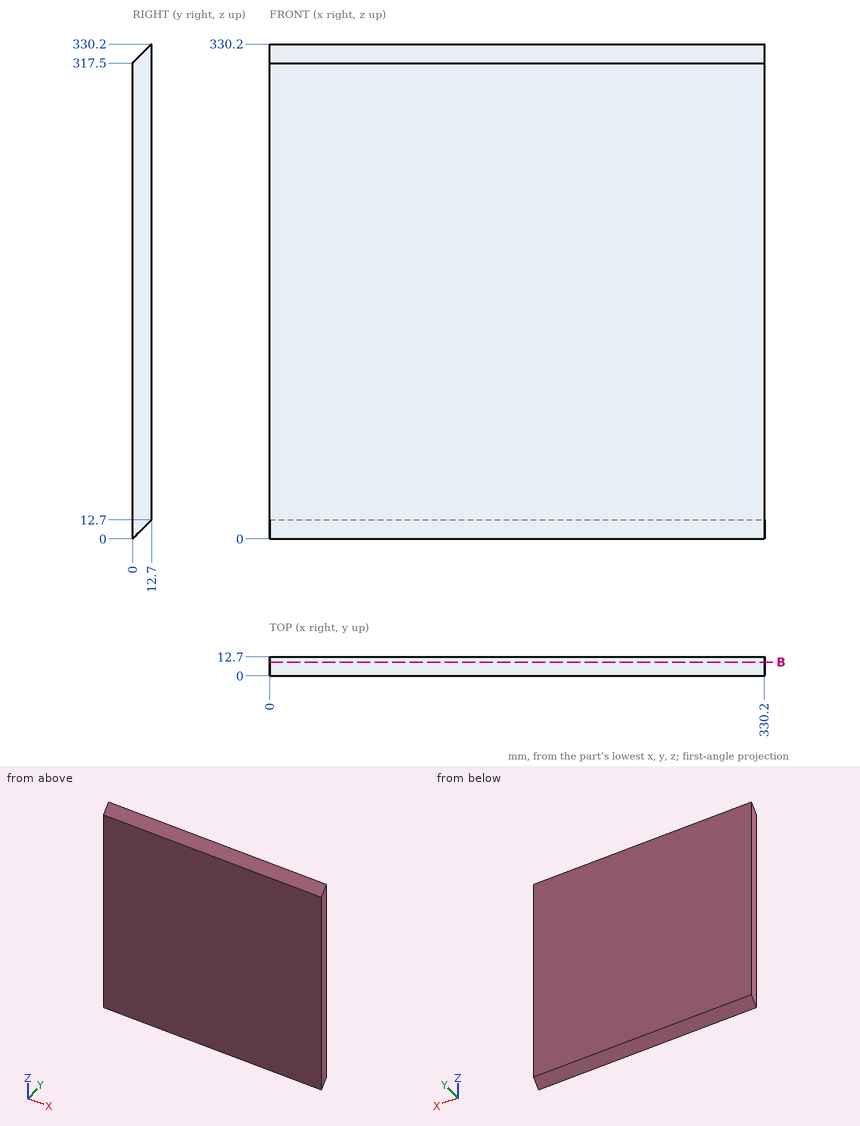
For this review, use the dimensioned drawing (mm, ordinates from the lowest corner) and the shaded views. Coordinates: 2 decimals unless noted, no trailing zeros. Order: outer loops, then holes, each group sorted by start corner. A loop starts at its lowest first (then second) coordinate and runs counter-clockwise, first axis right, second up. Notation, with made-up numbers: M 89.5,87.25 L 130.5,87.25 A23 cw 130.5,112.25 Z; hole C -16,35 d6. An arc over 180 degrees is marked long. Answer as a JSON object with one key per item and string values. Group by question number.
1) Wall thickness on L1, parallel to Z at x = 197, y = 9; L2, parallel to Z at x = 120.5, y = 11.25: over which ranges is each line inside the solid? List them lowest first.
2) For pin 1 (2 mm diameter, centred on x = 197.5, y = 5, fed in from -Z); pin 2 (1 mm diameter, centred on x = 250, y = 5.5, fed in from -Z), all flat-tipped, find the tip position at first contact; note any pin that passes through.
3) Add section B-B, the plane y = 9.25. Write out the cut boundary in (x, z), then the cut area to 3 significant figures.
Computed values:
{
 "1": {"L1": "z = 9 to 326.5", "L2": "z = 11.25 to 328.75"},
 "2": {"pin 1": "stops at z = 4", "pin 2": "stops at z = 5"},
 "3": {"outline": "M 0,9.25 L 330.2,9.25 L 330.2,326.75 L 0,326.75 Z", "area": "105,000 mm^2"}
}
